Verification items for the finished model (mm, model axes). Round coordinates to 2 decimals unless told otherwise and drop trailing zeros. Order: outer loops, then holes, each group sorted by start corner. A loop starts at its lowest first (then second) coordinate and runs counter-clockwise, first axis right, second up. Notation, with made-up numbers: M 39.5,-5 L 89.5,-5 A19 cw 89.5,32 Z; hole C 19,-26 d11. An arc over 180 degrees is marked long. Use one line per item in the form item = value. Start each with the question number.
Item 1: Cross-section at D-D on y = 72.5. Enter the section's corners in (x, z), then the cut area to 3 significant figures.
Item 2: Cross-section at B-B on y = 38. Enter the section's corners in (x, z).
Item 3: Cross-section at A-A on x = 99. Enter the section's corners in (y, z).
Item 4: Go/stop test with flat-tipped pins: pin 1 Ø1.2 at (x, z) = (3, 0.5) entering from -Y; pin 2 Ø1.2 at (x, z) = (91, 1) entering from -Y; pin 3 Ø0.8 at (y, z) = (52, 1) entering from +X. Record where each tip stops, or that it passes through.
Item 5: Cross-section at C-C on z = 0.9. Count the separate pieces of the cut face and the enclosed holes in it, then the cut area to 3 significant figures.
Item 6: Thickness scan on probe 1 along Y at (x, z) = (38.5, 0.2); probe 2 along Y at (x, z) = (-15, 1.75); probe 3 along X at (y, z) = (66, 1). Record the ranges inside material, lowest first. Write a range as [from, to].
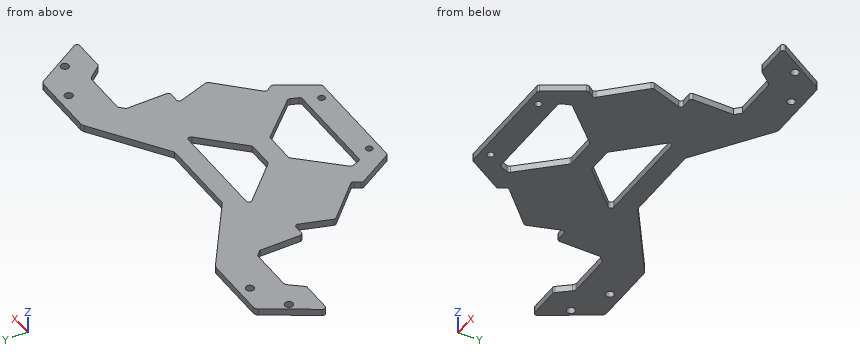
Autodesk Inventor part; units mm, degrees
ref_plane "YZ Plane" through (0, 0, 0) normal (1, 0, 0) x (0, 1, 0)
ref_plane "XZ Plane" through (0, 0, 0) normal (0, 1, 0) x (-1, 0, 0)
ref_plane "XY Plane" through (0, 0, 0) normal (0, 0, 1) x (1, 0, 0)
sketch "Sketch1" plane through (0, 0, 0) normal (0, 0, 1) x (1, 0, 0)
  line L0 (0, 76.5) -> (84, 76.5) construction
  line L1 (84, 76.5) -> (84, 0) construction
  line L2 (84, 0) -> (0, 0) construction
  line L3 (0, 0) -> (0, 76.5) construction
  line L4 (-37, 76.5) -> (0, 76.5) construction
  line L5 (0, 76.5) -> (0, 62) construction
  line L6 (0, 62) -> (-37, 62) construction
  line L7 (-37, 62) -> (-37, 76.5) construction
  line L8 (84, 76.5) -> (121, 76.5) construction
  line L9 (121, 76.5) -> (121, 62) construction
  line L10 (121, 62) -> (84, 62) construction
  line L11 (84, 62) -> (84, 76.5) construction
  line L12 (27, 58) -> (57, 58)
  line L13 (27, 58) -> (0.7665, 75.9748)
  line L14 (57, 58) -> (83.2335, 75.9748)
  line L15 (13.25, 14) -> (70.75, 14) construction
  line L16 (0, 76.5) -> (-25, 76.5) construction
  line L17 (-37, 76.5) -> (-37, 56.5) construction
  line L18 (-36.0913, 58.0145) -> (-25.5826, 75.529)
  line L19 (-35.2338, 56.5) -> (-23.9739, 56.5)
  line L20 (0, 62) -> (-19, 62) construction
  line L21 (-19.6002, 61.2665) -> (-23.1999, 56.8668)
  line L22 (0, 44) -> (84, 44) construction
  line L23 (1, 44) -> (4.371, 44)
  line L24 (83, 44) -> (79.629, 44)
  line L25 (1.5, 31) -> (82.5, 31) construction
  line L26 (5.3215, 42.6893) -> (1.6893, 31.579)
  line L27 (78.6785, 42.6893) -> (82.3107, 31.579)
  line L28 (15.3, 17) -> (68.7, 17) construction
  line L29 (82.0724, 30.5662) -> (69.278, 17.5864)
  line L30 (1.9276, 30.5662) -> (14.722, 17.5864)
  line L31 (69.1645, 16.3202) -> (70.3916, 14.5245)
  line L32 (14.8355, 16.3202) -> (13.6084, 14.5245)
  line L33 (21.5, 0) -> (62.5, 0) construction
  line L34 (21.2099, 0.4923) -> (13.5725, 13.4527)
  line L35 (62.7901, 0.4923) -> (70.4275, 13.4527)
  line L36 (84, 76.5) -> (109, 76.5) construction
  line L37 (121, 76.5) -> (121, 56.5) construction
  line L38 (120.0913, 58.0145) -> (109.5826, 75.529)
  line L39 (119.2338, 56.5) -> (107.9739, 56.5)
  line L40 (84, 62) -> (103, 62) construction
  line L41 (103.6002, 61.2665) -> (107.1999, 56.8668)
  line L42 (-23.8676, 76.5) -> (-0.9292, 76.5)
  line L43 (84.9292, 76.5) -> (107.8676, 76.5)
  line L44 (-18.0522, 62) -> (-2, 62)
  line L45 (102.0522, 62) -> (86, 62)
  line L46 (0, 60) -> (0, 45)
  line L47 (84, 60) -> (84, 45)
  line L48 (22.0714, 0) -> (61.9286, 0)
  line L49 (23.861, 51) -> (60.139, 51)
  line L50 (37.4235, 35) -> (46.5765, 35)
  line L51 (47.2947, 35.3042) -> (60.8572, 49.3042)
  line L52 (36.7053, 35.3042) -> (23.1428, 49.3042)
  line L53 (36.4346, 28) -> (47.5654, 28)
  line L54 (22, 13) -> (62, 13) construction
  line L55 (24.193, 9) -> (59.807, 9)
  line L56 (60.7433, 9.6489) -> (61.7824, 12.4197)
  line L57 (61.5771, 13.4531) -> (48.2965, 27.6823)
  line L58 (35.7035, 27.6823) -> (22.4229, 13.4531)
  line L59 (22.2176, 12.4197) -> (23.2567, 9.6489)
  line L60 (-28.5, 66) -> (112.5, 66) construction
  line L61 (-15, 72.5) -> (99, 72.5) construction
  line L62 (27, 3.5) -> (57, 3.5) construction
  arc A0 (0.7665, 75.9748) -> (-0.9292, 76.5) centre (-0.9292, 73.5) ccw
  arc A1 (84.9292, 76.5) -> (83.2335, 75.9748) centre (84.9292, 73.5) ccw
  arc A2 (-23.8676, 76.5) -> (-25.5826, 75.529) centre (-23.8676, 74.5) ccw
  arc A3 (109.5826, 75.529) -> (107.8676, 76.5) centre (107.8676, 74.5) ccw
  arc A4 (119.2338, 56.5) -> (120.0913, 58.0145) centre (119.2338, 57.5) ccw
  arc A5 (-36.0913, 58.0145) -> (-35.2338, 56.5) centre (-35.2338, 57.5) ccw
  arc A6 (-23.9739, 56.5) -> (-23.1999, 56.8668) centre (-23.9739, 57.5) ccw
  arc A7 (107.1999, 56.8668) -> (107.9739, 56.5) centre (107.9739, 57.5) ccw
  arc A8 (103.6002, 61.2665) -> (102.0522, 62) centre (102.0522, 60) ccw
  arc A9 (-18.0522, 62) -> (-19.6002, 61.2665) centre (-18.0522, 60) ccw
  line L63 (-2, 62) -> (0, 60)
  line L64 (84, 60) -> (86, 62)
  arc A10 (0, 45) -> (1, 44) centre (1, 45) ccw
  arc A11 (83, 44) -> (84, 45) centre (83, 45) ccw
  arc A12 (79.629, 44) -> (78.6785, 42.6893) centre (79.629, 43) ccw
  arc A13 (5.3215, 42.6893) -> (4.371, 44) centre (4.371, 43) ccw
  arc A14 (1.6893, 31.579) -> (1.9276, 30.5662) centre (2.6398, 31.2682) ccw
  arc A15 (82.0724, 30.5662) -> (82.3107, 31.579) centre (81.3602, 31.2682) ccw
  arc A16 (69.278, 17.5864) -> (69.1645, 16.3202) centre (69.9902, 16.8844) ccw
  arc A17 (70.4275, 13.4527) -> (70.3916, 14.5245) centre (69.5659, 13.9603) ccw
  arc A18 (61.9286, 0) -> (62.7901, 0.4923) centre (61.9286, 1) ccw
  arc A19 (21.2099, 0.4923) -> (22.0714, 0) centre (22.0714, 1) ccw
  arc A20 (13.6084, 14.5245) -> (13.5725, 13.4527) centre (14.4341, 13.9603) ccw
  arc A21 (14.8355, 16.3202) -> (14.722, 17.5864) centre (14.0098, 16.8844) ccw
  arc A22 (23.2567, 9.6489) -> (24.193, 9) centre (24.193, 10) ccw
  arc A23 (22.4229, 13.4531) -> (22.2176, 12.4197) centre (23.154, 12.7708) ccw
  arc A24 (36.4346, 28) -> (35.7035, 27.6823) centre (36.4346, 27) ccw
  arc A25 (48.2965, 27.6823) -> (47.5654, 28) centre (47.5654, 27) ccw
  arc A26 (61.7824, 12.4197) -> (61.5771, 13.4531) centre (60.846, 12.7708) ccw
  arc A27 (59.807, 9) -> (60.7433, 9.6489) centre (59.807, 10) ccw
  arc A28 (23.861, 51) -> (23.1428, 49.3042) centre (23.861, 50) ccw
  arc A29 (60.8572, 49.3042) -> (60.139, 51) centre (60.139, 50) ccw
  arc A30 (46.5765, 35) -> (47.2947, 35.3042) centre (46.5765, 36) ccw
  arc A31 (36.7053, 35.3042) -> (37.4235, 35) centre (37.4235, 36) ccw
  circle A32 centre (-15, 72.5) radius 1.5
  circle A33 centre (-28.5, 66) radius 1.5
  circle A34 centre (112.5, 66) radius 1.5
  circle A35 centre (99, 72.5) radius 1.5
  circle A36 centre (57, 3.5) radius 1.25
  circle A37 centre (27, 3.5) radius 1.25
  point P0 (-23.5, 56.5)
  point P1 (5.75, 44)
  point P2 (78.25, 44)
  point P3 (107.5, 56.5)
  point P4 (21.5, 51)
  point P5 (62.5, 51)
  point P6 (37, 35)
  point P7 (47, 35)
  point P8 (36, 28)
  point P9 (48, 28)
  point P10 (23.5, 9)
  point P11 (60.5, 9)
  dimension "d0" = 84
  dimension "d1" = 76.5
  dimension "d2" = 37
  dimension "d3" = 14.5
  dimension "d4" = 14.5
  dimension "d5" = 37
  dimension "d7" = 30
  dimension "d8" = 27
  dimension "d9" = 58
  dimension "d10" = 57.5
  dimension "d11" = 13.25
  dimension "d12" = 14
  dimension "d13" = 25
  dimension "d14" = 20
  dimension "d15" = 13.5
  dimension "d16" = 19
  dimension "d17" = 18
  dimension "d18" = 5.75
  dimension "d19" = 5.75
  dimension "d20" = 81
  dimension "d21" = 13
  dimension "d22" = 1.5
  dimension "d23" = 53.4
  dimension "d24" = 14
  dimension "d25" = 15.3
  dimension "d26" = 41
  dimension "d27" = 21.5
  dimension "d28" = 25
  dimension "d29" = 20
  dimension "d30" = 13.5
  dimension "d31" = 19
  dimension "d32" = 41
  dimension "d33" = 21.5
  dimension "d34" = 7
  dimension "d35" = 10
  dimension "d36" = 23
  dimension "d37" = 37
  dimension "d38" = 12
  dimension "d39" = 28
  dimension "d40" = 36
  dimension "d41" = 40
  dimension "d42" = 13
  dimension "d43" = 22
  dimension "d44" = 37
  dimension "d45" = 9
  dimension "d46" = 23.5
  dimension "d47" = 141
  dimension "d48" = 10.5
  dimension "d49" = 8.5
  dimension "d50" = 114
  dimension "d51" = 4
  dimension "d52" = 22
  dimension "d53" = 30
  dimension "d54" = 3.5
  dimension "d55" = 27
  dimension "d56" = 3
  dimension "d57" = 3
  dimension "d58" = 2
  dimension "d59" = 2
  dimension "d60" = 1
  dimension "d61" = 1
  dimension "d62" = 1
  dimension "d63" = 1
  dimension "d64" = 2
extrude "Extrusion2" add sketch "Sketch1" along normal blind 2.5
properties part number "RCT-H001_Al_side_plate"
Output values:
q1.outline = M -27.4,0 L -16.5,0 L -16.5,2.5 L -27.4,2.5 Z; M -13.5,0 L 5.84,0 L 5.84,2.5 L -13.5,2.5 Z; M 78.16,0 L 97.5,0 L 97.5,2.5 L 78.16,2.5 Z; M 100.5,0 L 111.4,0 L 111.4,2.5 L 100.5,2.5 Z
q1.area = 151 mm2
q2.outline = M 3.79,0 L 34.09,0 L 34.09,2.5 L 3.79,2.5 Z; M 49.91,0 L 80.21,0 L 80.21,2.5 L 49.91,2.5 Z
q3.outline = M 62,0 L 71,0 L 71,2.5 L 62,2.5 Z; M 74,0 L 76.5,0 L 76.5,2.5 L 74,2.5 Z
q4.pin_1 = 28.87
q4.pin_2 = 62
q4.pin_3 = 84
q5.separate_pieces = 1
q5.enclosed_holes = 8
q5.area = 4,490 mm2
q6.probe_1 = [0, 9], [28, 35], [51, 58]
q6.probe_2 = [62, 71], [74, 76.5]
q6.probe_3 = [-31.3, -30], [-27, 15.32], [68.68, 111], [114, 115.3]
